For this review, use the dimensioned drawing (mm, ordinates from the lowest corner) and the shaded views. Give positions to 0.01 mm unless a question says otherwise; leave off trailing zeros. Loops run counter-clockwise (first coordinate to the right, second up) from the corner with the lowest first, then second, coordinate; pieces in that order, holes last. Notation, with made-up numbers: M 67,-17 L 114,-17 A37 cw 114,19 Z; hole C 72,48 d4. An arc over 180 degrees is marked long. Use a Markdown table: item, result. Add a question column.
(1) Draft analysis for pull direction X (two halves, no side actions). For the marked faces 1, 2, 3 and 4, state which applies: pulls with the +X half, pulls with the -X half, needs draft (parallel to the pull), parting line crosses it, or undercut.
(2) Add section D-D, the plane z = 1.75. Give the boundary of the cut face in (x, y).
(3) For probe 1 along Z at (x, y) = (5, 8); probe 2 along Y at (x, z) = (43, 9); probe 3 along X at (y, z) = (6.5, 4.25), list the stretches that pass through material, from the lowest coordinate up.
(4) Add section B-B, the plane x = 60. Give the boundary of the cut face in (y, z), then the cut area to 3 significant figures.
(5) Add section A-A, the plane y = 9.5. Give the boundary of the cut face in (x, z).
(6) Add section C-C, the plane y = 6.5. Give the boundary of the cut face in (x, z), then the cut area to 3 significant figures.
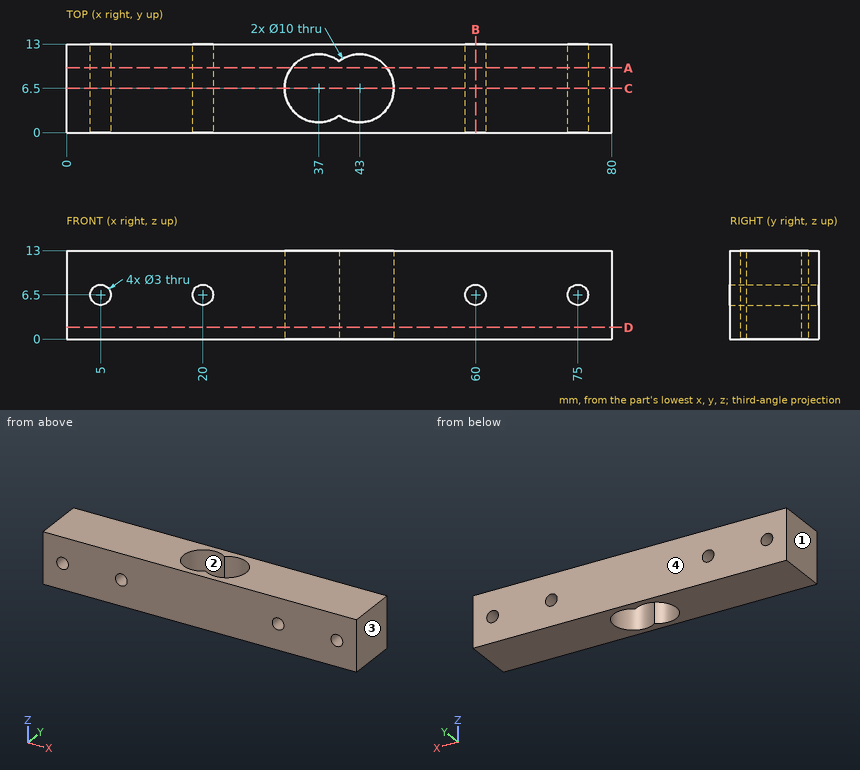
Established:
| question | item | result |
|---|---|---|
| 1 | face 1 | pulls with the -X half |
| 1 | face 2 | undercut |
| 1 | face 3 | pulls with the +X half |
| 1 | face 4 | needs draft |
| 2 | outline | M 0,0 L 80,0 L 80,13 L 0,13 Z; hole M 40,2.5 A5 ccw long 40,10.5 A5 ccw long Z |
| 3 | probe 1 | 0 to 5, 8 to 13 |
| 3 | probe 2 | 0 to 1.5, 11.5 to 13 |
| 3 | probe 3 | 0 to 32, 48 to 80 |
| 4 | outline | M 0,0 L 13,0 L 13,5 L 0,5 Z; M 0,8 L 13,8 L 13,13 L 0,13 Z |
| 4 | area | 130 mm^2 |
| 5 | outline | M 0,0 L 33,0 L 33,13 L 0,13 Z; M 47,0 L 80,0 L 80,13 L 47,13 Z; hole C 5,6.5 d3; hole C 20,6.5 d3; hole C 60,6.5 d3; hole C 75,6.5 d3 |
| 6 | outline | M 0,0 L 32,0 L 32,13 L 0,13 Z; M 48,0 L 80,0 L 80,13 L 48,13 Z; hole C 5,6.5 d3; hole C 20,6.5 d3; hole C 60,6.5 d3; hole C 75,6.5 d3 |
| 6 | area | 804 mm^2 |
